Input: part model. Units: mm. Frame: model coordinates. Give positions to 0.01 mm unless a question says otherwise; leave off trailing zeros. Order: outer loops, then holes, each group sorted by start corner. A loop starts at its lowest first (then second) coordinate and runs counter-clockwise, first axis right, second up. Notation, with made-up numbers: M 0.5,-15 L 17.5,-15 A28 ccw 17.5,15 Z; hole C -31.5,89 d4. An arc over 180 degrees is marked long. Use a Markdown table: item, result.
Autodesk Inventor part; units mm, degrees
ref_plane "YZ Plane" through (0, 0, 0) normal (1, 0, 0) x (0, 1, 0)
ref_plane "XZ Plane" through (0, 0, 0) normal (0, 1, 0) x (-1, 0, 0)
ref_plane "XY Plane" through (0, 0, 0) normal (0, 0, 1) x (1, 0, 0)
sketch "Эскиз1" plane through (0, 0, 0) normal (0, 1, 0) x (-1, 0, 0)
  line L0 (0, 0) -> (400, 0)
  line L1 (400, 0) -> (400, -400)
  line L2 (400, -400) -> (0, -400)
  line L3 (0, -400) -> (0, 0)
  dimension "d0" = 400
  dimension "d1" = 400
extrude "Выдавливание1" add sketch "Эскиз1" along normal blind 6
sketch "Эскиз2" plane through (0, 6, 0) normal (0, 1, 0) x (1, 0, 0)
  circle A0 centre (-203, 203) radius 25
  line L0 (-400, 0) -> (0, 0)
  line L1 (0, 0) -> (0, 400)
  dimension "d4" = 50
  dimension "d5" = 203
  dimension "d6" = 203
extrude "Выдавливание2" cut sketch "Эскиз2" against normal blind 6
sketch "Эскиз3" plane through (0, 6, 0) normal (0, 1, 0) x (1, 0, 0)
  line L0 (-400, 0) -> (0, 0)
  line L1 (0, 0) -> (-3, 0)
  line L2 (-3, 0) -> (-3, 3)
  line L3 (-3, 3) -> (0, 3)
  line L4 (0, 3) -> (0, 0)
  line L5 (0, 0) -> (0, 400)
  line L6 (0, 400) -> (-3, 400)
  line L7 (-3, 400) -> (-3, 397)
  line L8 (-3, 397) -> (0, 397)
  line L9 (0, 397) -> (0, 400)
  line L10 (-400, 400) -> (-400, 0)
  line L11 (-400, 400) -> (-397, 400)
  line L12 (-397, 400) -> (-397, 397)
  line L13 (-397, 397) -> (-400, 397)
  line L14 (-400, 397) -> (-400, 400)
  line L15 (-400, 0) -> (-397, 0)
  line L16 (-397, 0) -> (-397, 3)
  line L17 (-397, 3) -> (-400, 3)
  line L18 (-400, 3) -> (-400, 0)
  point P0 (0, 397)
  point P1 (-400, 3)
  point P2 (-397, 0)
  dimension "d9" = 3
  dimension "d10" = 3
  dimension "d11" = 3
  dimension "d12" = 3
  dimension "d13" = 3
  dimension "d14" = 3
  dimension "d15" = 3
properties part number "Днище"
1) First-contact query: pin 1 Ø4 at (x, z) = (-100.5, -154) entering from -Y. Flat tip, straight axial feed; report the tip coordinate or a pass-through.
Response values:
| item | result |
|---|---|
| pin 1 | stops at y = 0 |
2) Cut plane A-A on x = -203. Return loops of the section in (y, z), and give its area (3 significant figures).
Response values:
| item | result |
|---|---|
| outline | M 0,-400 L 6,-400 L 6,-228 L 0,-228 Z; M 0,-178 L 6,-178 L 6,0 L 0,0 Z |
| area | 2,100 mm² |
3) Material intervals for line 1 (X direction, y = 1.5, z = -203); line 2 (X direction, y = 4.15, z = -208), sorted ascending. Write a range as from..to.
Response values:
| item | result |
|---|---|
| line 1 | x = -400..-228, -178..0 |
| line 2 | x = -400..-227.49, -178.51..0 |
4) Mould query, pull axis Z, two halves, no side actions, for faces 1 (the face through (-153, 6, -197)), 2 (the face through (-189.56, 3.04, -224.08)). Classes: released by +Z, released by -Z, zero draft, split by the parting line, or undercut.
Response values:
| item | result |
|---|---|
| face 1 | zero draft |
| face 2 | undercut |
5) Cut plane B-B on z = -203. Return loops of the section in (x, y).
Response values:
| item | result |
|---|---|
| outline | M -400,0 L -228,0 L -228,6 L -400,6 Z; M -178,0 L 0,0 L 0,6 L -178,6 Z |
